Autodesk Inventor part; units mm, degrees
ref_plane "YZ Plane" through (0, 0, 0) normal (1, 0, 0) x (0, 1, 0)
ref_plane "XZ Plane" through (0, 0, 0) normal (0, 1, 0) x (-1, 0, 0)
ref_plane "XY Plane" through (0, 0, 0) normal (0, 0, 1) x (1, 0, 0)
sketch "Sketch1" plane through (0, 0, 0) normal (0, 1, 0) x (-1, 0, 0)
  line L0 (0, 0) -> (30, 0)
  line L1 (30, 0) -> (30, -60)
  line L2 (30, -60) -> (0, -60)
  line L3 (0, -60) -> (0, 0)
  dimension "d0" = 30
  dimension "d1" = 60
extrude "Extrusion1" add sketch "Sketch1" along normal blind 1.7272
sketch "Sketch2" plane through (-30, 0, 0) normal (0, 0, 1) x (1, 0, 0)
  line L0 (30, 0) -> (0, 0)
  line L1 (5.475, 0) -> (24.525, 0)
  line L2 (24.525, 0) -> (24.525, 6.7272)
  line L3 (24.525, 6.7272) -> (5.475, 6.7272)
  line L4 (5.475, 6.7272) -> (5.475, 0)
  point P0 (15, 6.7272)
  point P1 (15, 0)
  dimension "d4" = 19.05
  dimension "d5" = 6.7272
extrude "Extrusion2" add sketch "Sketch2" along normal blind 1.7272
sketch "Sketch3" plane through (-30, 0, 0) normal (0, 0, -1) x (-1, 0, 0)
  line L0 (-24.525, 6.7272) -> (-5.475, 6.7272)
  line L1 (-5.475, 6.7272) -> (-5.475, 1.7272)
  line L2 (-24.525, 6.7272) -> (-5.475, 6.7272)
  line L3 (-5.475, 6.7272) -> (-5.475, 5)
  line L4 (-5.475, 5) -> (-24.525, 5)
  line L5 (-24.525, 5) -> (-24.525, 6.7272)
  point P0 (-30, 0)
  dimension "d8" = 1.7272
extrude "Extrusion3" add sketch "Sketch3" along normal blind 3.175
sketch "Sketch4" plane through (0, 0, -60) normal (0, 0, -1) x (-1, 0, 0)
  line L0 (30, 0) -> (0, 0)
  line L1 (5.475, 6.7272) -> (24.525, 6.7272)
  line L2 (24.525, 6.7272) -> (24.525, 0)
  line L3 (24.525, 0) -> (5.475, 0)
  line L4 (5.475, 0) -> (5.475, 6.7272)
  line L5 (24.525, 6.7272) -> (5.475, 6.7272)
  point P0 (15, 6.7272)
  point P1 (15, 6.7272)
  dimension "d11" = 19.05
  dimension "d12" = 6.7272
extrude "Extrusion4" add sketch "Sketch4" along normal blind 1.7272
sketch "Sketch5" plane through (0, 0, -60) normal (0, 0, 1) x (1, 0, 0)
  line L0 (-5.475, 6.7272) -> (-24.525, 6.7272)
  line L1 (-5.475, 1.7272) -> (-5.475, 6.7272)
  line L2 (-24.525, 6.7272) -> (-5.475, 6.7272)
  line L3 (-5.475, 6.7272) -> (-5.475, 5)
  line L4 (-5.475, 5) -> (-24.525, 5)
  line L5 (-24.525, 5) -> (-24.525, 6.7272)
  point P0 (0, 0)
  dimension "d15" = 1.7272
extrude "Extrusion5" add sketch "Sketch5" along normal blind 3.175
chamfer "Chamfer1" distance 1.7272 angle 45 2 edges at (-15, 5, -3.175) (-15, 5, -56.825)
properties part number "PanelHolder"
CAD build for the part. Positions are in the model's coordinates, mm. A direction names the side the tool comes from. Give positions to 0.01 mm unless a question says otherwise; leave off trailing zeros. Loops run counter-clockwise (first coordinate to the right, second up) from the corner with the lowest first, then second, coordinate; pieces in that order, holes last. Notation, with made-up numbers: M 61,80 L 72,80 A28 ccw 72,109 Z; hole C -7,26.25 d8. An arc over 180 degrees is marked long. Write each question's results on one line, items separated by ' | '.
Q1. Band-saw the part on C-C on z = -39. Write the cut outline in (x, y), and give its area (3 significant figures).
Geometry check:
outline: M -30,0 L 0,0 L 0,1.73 L -30,1.73 Z | area: 51.8 mm²
Q2. Band-saw the part on A-A on y = 3. Write the cut outline in (x, z) (3 decimals).
Geometry check:
outline: M -24.525,-61.727 L -5.475,-61.727 L -5.475,-60 L -24.525,-60 Z; M -24.525,0 L -5.475,0 L -5.475,1.727 L -24.525,1.727 Z
Q3. Which spindle directions (+Z, -Z, +X, -X, +Y, -Y) get a long thin tool onto all of the face, cutting with end or side? Do faces 4 (the face through (-5.475, 4.1, 0.4)), 5 (the face through (-3, 1, 0)), 6 (the face through (-15, 5, -1)). Say none if no direction does.
Geometry check:
face 4: +Z, +X, +Y | face 5: +Z, +X, +Y, -Y | face 6: +X, -X
Q4. Band-saw the part on D-D on x = -25.25. Write the cut outline in (y, z), and give its area (3 significant figures).
Geometry check:
outline: M 0,-60 L 1.73,-60 L 1.73,0 L 0,0 Z | area: 104 mm²
Q5. Mould opens along Z. For faces 1 (the face through (-15, 6.727, -1)), 2 (the face through (-15, 5, -59)), 3 (the face through (-15, 3, 1.727)) say: pulls with the +Z half, pulls with the -Z half, needs draft (parallel to the pull), parting line crosses it, or undercut.
Geometry check:
face 1: needs draft | face 2: undercut | face 3: pulls with the +Z half
Q6. Flat gauge pins, fed straight in: P1, Ø4, axis at y = 4.5, z = -20, coming from the +X side; P2, Ø4, axis at y = 4, z = -0.5, coming from the -X side (3 decimals); P3, Ø1.4, axis at x = -28, y = 1, coming from the -Z side; P4, Ø9, axis at x = -21.5, z = -17.5, coming from the +Y side. Where does each tip first touch, or does it go through?
Geometry check:
P1: passes through | P2: stops at x = -24.525 | P3: stops at z = -60 | P4: stops at y = 1.73
Q7. Probe probe 1 along Z at (x, y) = (-11, 4.25); probe 2 along Z at (x, y) = (-6, 6); probe 3 along Y at (x, z) = (-16.75, -38). List the from-to ranges inside material, lowest first.
Geometry check:
probe 1: z = -61.73 to -60, 0 to 1.73 | probe 2: z = -61.73 to -57.55, -2.45 to 1.73 | probe 3: y = 0 to 1.73
